Part model, mm, in its own coordinate system. Face numbers are marked on the shaded views. A direction names the side the tool comes from. Coordinates: 2 decimals unless noted, no trailing zeros. Loops run counter-clockwise (first coordinate to the right, second up) from the corner with the lowest first, then second, coordinate; pieces in that order, holes last. Notation, with made-up numbers: (-29, -30.5) -> (28, -30.5) arc R25 cw to (28, -9.5) -> close; hole circle Ø7 at (59.5, -30). An arc over 180 degrees is marked (long way). One line per question, with ' | ' between items. Start each with the question number.
1) Cut at D-D (x = -1). List the corners of the cut face in (y, z).
2) Cut at B-B (z = 0). List the corners of the cut face in (x, y), plus the area to 3 significant figures.
3) Probe L1, parallel to X at y = 4.75, z = 0; L2, parallel to Y at x = 1.5, z = -1.25; L3, parallel to X at y = 9.5, z = 2.25. List the from-to ranges inside material, lowest first. Write a range as from..to.
4) Cut at C-C (y = 10.5). List the corners of the cut face in (x, z), plus the area to 3 significant figures.
5) 3-axis set-ups, long thin cutter, end or side, ignore diameter. For the marked faces 4 and 5: which of +Z, -Z, +X, -X, +Y, -Y reach the whole face in a straight line?
6) Drop flat-ended pins along their axis: pin 1 (1 mm diameter, centred on x = -3, y = 7, fed in from +Z); pin 2 (3 mm diameter, centred on y = 14.5, z = 4, fed in from +X); pin 3 (1 mm diameter, centred on x = -0.5, z = -0.5, fed in from -Y). Give the stop position or say it passes through.
7) Two-plate mould, pull along X, no slides. Class the marked faces 1, 2 and 3: released by +X, released by -X, zero draft, split by the parting line, or undercut.
8) Cut at A-A (y = 5.25). List the corners of the cut face in (x, z), plus the area to 3 significant figures.
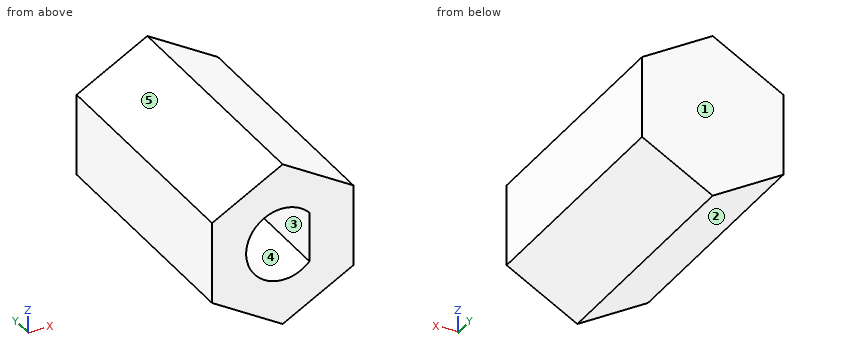
from build123d import *

# Parameters (mm, degrees)
BOSS_EXTRUDE1_DEPTH = 19.05
CUT_EXTRUDE1_DEPTH  = 10.16


with BuildPart() as part:
    # Sketch1 → Boss-Extrude1 (new body)
    with BuildSketch(Plane(origin=(0, 0, 0), x_dir=(1, 0, 0), z_dir=(0, 1, 0))):
        Polygon((-5.279290861, -3.048), (0, -6.096), (5.279290861, -3.048), (5.279290861, 3.048), (0, 6.096), (-5.279290861, 3.048), align=None)
    extrude(amount=BOSS_EXTRUDE1_DEPTH)

    # Sketch1_3 → Cut-Extrude1 (cut)
    with BuildSketch(Plane(origin=(0, 0, 0), x_dir=(1, 0, 0), z_dir=(0, 1, 0))):
        with BuildLine():
            Line((2, -1.858932557), (2, 1.858932557))
            ThreePointArc((2, 1.858932557), (-2.7305, 0), (2, -1.858932557))
        make_face()
    extrude(amount=CUT_EXTRUDE1_DEPTH, mode=Mode.SUBTRACT)


solid = part.part
Reported:
1) outline: (0, -5.52) -> (19.05, -5.52) -> (19.05, 5.52) -> (0, 5.52) -> (0, 2.54) -> (10.16, 2.54) -> (10.16, -2.54) -> (0, -2.54) -> close
2) outline: (-5.28, 0) -> (-2.73, 0) -> (-2.73, 10.16) -> (2, 10.16) -> (2, 0) -> (5.28, 0) -> (5.28, 19.05) -> (-5.28, 19.05) -> close | area: 153 mm²
3) L1: x = -5.28..-2.73, 2..5.28 | L2: y = 10.16..19.05 | L3: x = -5.28..-1.55, 1.55..5.28
4) outline: (-5.28, -3.05) -> (0, -6.1) -> (5.28, -3.05) -> (5.28, 3.05) -> (0, 6.1) -> (-5.28, 3.05) -> close | area: 96.5 mm²
5) face 4: -Y | face 5: +Z, -X, +Y, -Y
6) pin 1: stops at z = 4.65 | pin 2: stops at x = 5.28 | pin 3: stops at y = 10.16
7) face 1: zero draft | face 2: released by -X | face 3: undercut
8) outline: (-5.28, -3.05) -> (0, -6.1) -> (5.28, -3.05) -> (5.28, 3.05) -> (0, 6.1) -> (-5.28, 3.05) -> close; hole (2, -1.86) -> (2, 1.86) arc R2.73 ccw (long way) to start | area: 75.0 mm²
